Could you check a few things on this model? Use its own coordinates, in mm. Give positions to 0.01 mm unless a question says otherwise; leave off trailing zeros. Loops run counter-clockwise (first coordinate to the right, second up) from the corner with the lowest first, then second, coordinate; pieces in that order, holes last. Notation, with made-up numbers: (-1.75, -17.5) -> (19.25, -17.5) arc R22 cw to (19.25, 9.5) -> close; hole circle Ø4 at (70, 20). An arc over 180 degrees is marked (long way). Put each result on its own line as item: value.
```python
from build123d import *

# Parameters (mm, degrees)
SKETCH_1_W          = 9
SKETCH_1_H          = 6.5
EXTRUDE_1_DEPTH     = 200
SKETCH_2_R          = 1.75
CUT_EXTRUDE_2_DEPTH = 8
SKETCH_3_R          = 3
CUT_EXTRUDE_3_DEPTH = 3.5
CHAMFER_1_SIZE      = 0.5


with BuildPart() as part:
    # 草图1 → 拉伸1 (new body)
    with BuildSketch(Plane(origin=(0, 0, 0), x_dir=(0, 0, -1), z_dir=(1, 0, 0))):
        Rectangle(SKETCH_1_W, SKETCH_1_H)
    extrude(amount=EXTRUDE_1_DEPTH)

    # 草图2 → 拉伸2 (cut)
    with BuildSketch(Plane.XZ.offset(3.25)):
        with Locations(Location((10, 0, 0), (0, 0, 270))):
            Circle(SKETCH_2_R)
        with Locations(Location((170, 0, 0), (0, 0, 270))):
            Circle(SKETCH_2_R)
        with Locations(Location((190, 0, 0), (0, 0, 270))):
            Circle(SKETCH_2_R)
        with Locations((210, 0)):
            Circle(SKETCH_2_R)
        with Locations((230, 0)):
            Circle(SKETCH_2_R)
        with Locations((250, 0)):
            Circle(SKETCH_2_R)
        with Locations((270, 0)):
            Circle(SKETCH_2_R)
        with Locations((290, 0)):
            Circle(SKETCH_2_R)
        with Locations(Location((30, 0, 0), (0, 0, 270))):
            Circle(SKETCH_2_R)
        with Locations(Location((50, 0, 0), (0, 0, 270))):
            Circle(SKETCH_2_R)
        with Locations(Location((70, 0, 0), (0, 0, 270))):
            Circle(SKETCH_2_R)
        with Locations(Location((90, 0, 0), (0, 0, 270))):
            Circle(SKETCH_2_R)
        with Locations(Location((110, 0, 0), (0, 0, 270))):
            Circle(SKETCH_2_R)
        with Locations(Location((130, 0, 0), (0, 0, 270))):
            Circle(SKETCH_2_R)
        with Locations(Location((150, 0, 0), (0, 0, 270))):
            Circle(SKETCH_2_R)
    extrude(amount=-CUT_EXTRUDE_2_DEPTH, mode=Mode.SUBTRACT)

    # 草图3 → 拉伸3 (cut)
    with BuildSketch(Plane.XZ.offset(3.25)):
        with Locations(Location((10, 0, 0), (0, 0, 270))):
            Circle(SKETCH_3_R)
        with Locations(Location((170, 0, 0), (0, 0, 270))):
            Circle(SKETCH_3_R)
        with Locations(Location((190, 0, 0), (0, 0, 270))):
            Circle(SKETCH_3_R)
        with Locations((210, 0)):
            Circle(SKETCH_3_R)
        with Locations((230, 0)):
            Circle(SKETCH_3_R)
        with Locations((250, 0)):
            Circle(SKETCH_3_R)
        with Locations((270, 0)):
            Circle(SKETCH_3_R)
        with Locations((290, 0)):
            Circle(SKETCH_3_R)
        with Locations(Location((30, 0, 0), (0, 0, 270))):
            Circle(SKETCH_3_R)
        with Locations(Location((50, 0, 0), (0, 0, 270))):
            Circle(SKETCH_3_R)
        with Locations(Location((70, 0, 0), (0, 0, 270))):
            Circle(SKETCH_3_R)
        with Locations(Location((90, 0, 0), (0, 0, 270))):
            Circle(SKETCH_3_R)
        with Locations(Location((110, 0, 0), (0, 0, 270))):
            Circle(SKETCH_3_R)
        with Locations(Location((130, 0, 0), (0, 0, 270))):
            Circle(SKETCH_3_R)
        with Locations(Location((150, 0, 0), (0, 0, 270))):
            Circle(SKETCH_3_R)
    extrude(amount=-CUT_EXTRUDE_3_DEPTH, mode=Mode.SUBTRACT)

    # 倒角1
    chamfer_1_edges = [part.edges().sort_by_distance(p)[0] for p in [
        (100, 3.25, 4.5),
        (100, 3.25, -4.5),
        (100, -3.25, -4.5),
        (100, -3.25, 4.5),
    ]]
    chamfer(chamfer_1_edges, length=CHAMFER_1_SIZE)


solid = part.part
```
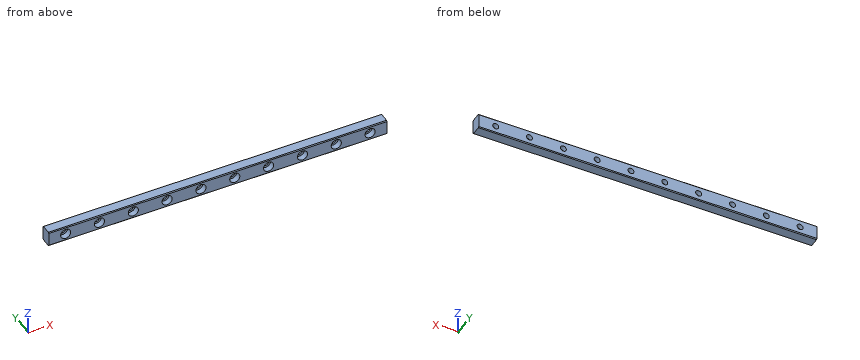
1. I need wall thicknesses on line 1 (Z direction, x = 150, y = 2.5); line 2 (Y direction, x = 171.5, z = -2). Which ranges of each line are inside material? Lowest first, please.
Recorded:
line 1: z = -4.5 to -1.75, 1.75 to 4.5
line 2: y = 0.25 to 3.25
2. I'm going to push a flat-ended pin straight in: pin 1 (2 mm diameter, centred on x = 70, z = 0, fed in from -Y). Where does the tip first touch, or does it pass through?
Recorded:
pin 1: passes through
3. If we section it at A-A (y = -1.5): Count the separate pieces of the cut face and the enclosed holes in it, then the cut area to 3 significant figures.
Recorded:
separate pieces: 1
enclosed holes: 10
area: 1,520 mm^2
4. If we section it at B-B (x = 90): List the corners of the cut face in (y, z) for me.
Recorded:
outline: (-3.25, -4) -> (-2.75, -4.5) -> (2.75, -4.5) -> (3.25, -4) -> (3.25, -1.75) -> (0.25, -1.75) -> (0.25, -3) -> (-3.25, -3) -> close; (-3.25, 3) -> (0.25, 3) -> (0.25, 1.75) -> (3.25, 1.75) -> (3.25, 4) -> (2.75, 4.5) -> (-2.75, 4.5) -> (-3.25, 4) -> close
